Design review of the part built by this model. Coordinates are the model's own, in mm. Face numbers are marked on the shaded views. A direction names the side the tool comes from. Coordinates: 2 decimals unless noted, no trailing zeros. Write each loop counter-clockwise with the first axis right and the second up, starting at its lowest first coordinate (ties: lowest second). Pieces come first, ordered by that corner, then holes. Notation, with made-up numbers: (-11.5, 86) - (29.5, 86) arc R12 cw to (29.5, 92) - close; hole circle Ø7 at (81, 25). An arc over 180 degrees is marked (long way). Answer as CSV lines item,"result". Start each with the question number.
Q1. We need section B-B (z = -5). Write out the cut boundary in (x, y).
Q2. Mouldability with a two-part tool opening along Y and no side actions: class the marked faces 3, 4 and 5 as pulls with the +Y half, pulls with the -Y half, needs draft (parallel to the pull), parting line crosses it, or undercut.
Q3. Clearance check with flat-ended pins moving along their axes: pin 1 (1 mm diameter, centred on x = -1, z = -1, fed in from -Y); pin 2 (2 mm diameter, centred on x = 0, y = 0, fed in from +Z); pin 3 (1.5 mm diameter, centred on y = -1, z = -5, fed in from -X). State where each tip first meets the part, or that it passes through.
Q4. For line 1 along Z through (x, y) = (-0.1, 0.55); line 2 along Z through (x, y) = (0.3, -1.95); line 3 along Y through (x, z) = (-1.3, 1), list the stretches that pass through material, from the lowest coordinate up. Write a range as [from, to].
Q5. We need section A-A (y = 0). Write out the cut boundary in (x, z) (3 decimals), plus the area to 3 significant figures.
Q6. Machinability: for the marked faces 1 and 2, which of the approach directions +Z, -Z, +X, -X, +Y, -Y give a long, thin tool a straight path to every point of the face, cutting with its end or side? Answer none if there is none.
from build123d import *

# Parameters (mm, degrees)
CUT_EXTRUDE1_DEPTH = 1.5
CHAMFER1_SIZE      = 0.15


with BuildPart() as part:
    # Sketch2 → Revolve1 (revolve)
    with BuildSketch(Plane(origin=(0, 0, 0), x_dir=(0, 0, -1), z_dir=(1, 0, 0)), mode=Mode.PRIVATE) as revolve1_sk:
        Polygon((-7.5, 0), (-7.5, 2.75), (-4.5, 2.75), (-4.5, 1.5), (7.125, 1.5), (7.5, 1.125), (7.5, 0), align=None)
    revolve(revolve1_sk.sketch.rotate(Axis((0, 0, 7.5), (0, 0, -1)), 90), axis=Axis((0, 0, 7.5), (0, 0, -1)))

    # Sketch3 → Cut-Extrude1 (cut)
    with BuildSketch(Plane.XY.offset(7.5)):
        Polygon((0, 1.443375673), (-1.25, 0.721687836), (-1.25, -0.721687836), (0, -1.443375673), (1.25, -0.721687836), (1.25, 0.721687836), align=None)
    extrude(amount=-CUT_EXTRUDE1_DEPTH, mode=Mode.SUBTRACT)

    # Cut-Extrude2 cone 1 section (through the dimple's axis) → Cut-Extrude2 (revolve, cut)
    with BuildSketch(Plane(origin=(0, 0, 7.5), x_dir=(0, -1, 0), z_dir=(1, 0, 0))):
        Polygon((0, 0), (1.443375673, 0), (0, 1.443375673), align=None)
    revolve(axis=Axis((0, 0, 7.5), (0, 0, -1)), mode=Mode.SUBTRACT)

    # Chamfer1
    chamfer1_edges = [part.edges().sort_by_distance(p)[0] for p in [
        (-2.75, 0, 4.5),
        (-2.75, 0, 7.5),
    ]]
    chamfer(chamfer1_edges, length=CHAMFER1_SIZE)


solid = part.part
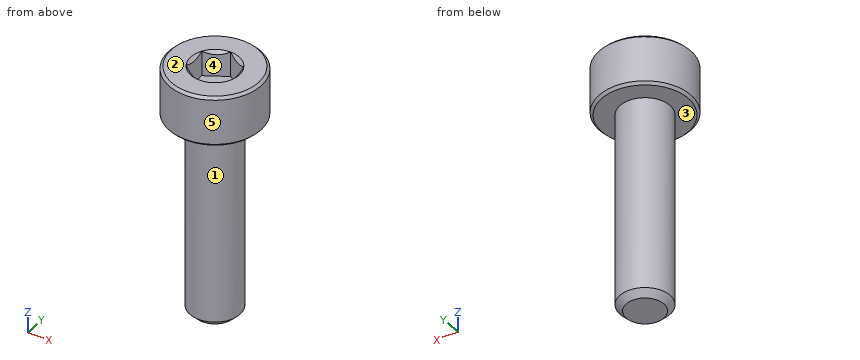
Results list:
1,outline,"circle Ø3 at (0, 0)"
2,face 3,"needs draft"
2,face 4,"undercut"
2,face 5,"parting line crosses it"
3,pin 1,"stops at y = -1.41"
3,pin 2,"stops at z = 6"
3,pin 3,"stops at x = -1.48"
4,line 1,"z = [-7.5, 6]"
4,line 2,"z = [4.5, 7.5]"
4,line 3,"y = [-0.75, 0.75]"
5,outline,"(-2.75, 4.65) - (-2.6, 4.5) - (-1.5, 4.5) - (-1.5, -7.125) - (-1.125, -7.5) - (1.125, -7.5) - (1.5, -7.125) - (1.5, 4.5) - (2.6, 4.5) - (2.75, 4.65) - (2.75, 7.35) - (2.6, 7.5) - (1.443, 7.5) - (1.25, 7.307) - (1.25, 6) - (-1.25, 6) - (-1.25, 7.307) - (-1.443, 7.5) - (-2.6, 7.5) - (-2.75, 7.35) - close"
5,area,"48.5 mm2"
6,face 1,"-Z"
6,face 2,"+Z, +X, -X, +Y, -Y"
